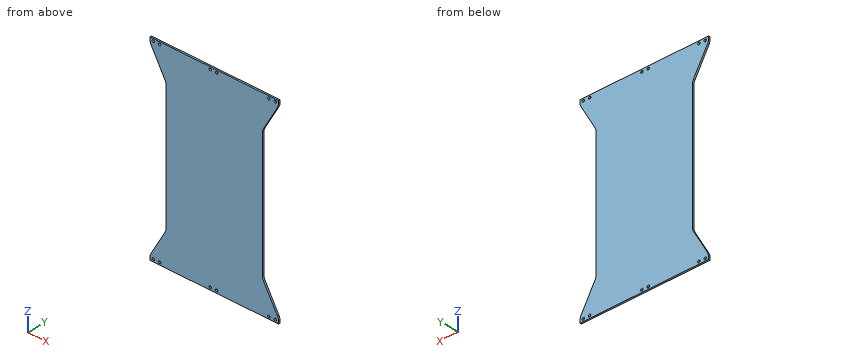
from build123d import *

# Parameters (mm, degrees)
SKETCH2_R           = 1.5
BOSS_EXTRUDE1_DEPTH = 2
FILLET1_R           = 10


with BuildPart() as part:
    # Sketch2 → Boss-Extrude1 (new body)
    with BuildSketch(Plane(origin=(0, 0, 0), x_dir=(1, 0, 0), z_dir=(0, 1, 0))):
        Polygon((688.047893911, -1476.918579287), (688.047893911, -1482.918579287), (708.047893911, -1517.918579287), (708.047893911, -1677.918579287), (688.047893911, -1712.918579287), (688.047893911, -1718.918579287), (847.682893911, -1718.918579287), (847.682893911, -1712.918579287), (827.682893911, -1677.918579287), (827.682893911, -1517.918579287), (847.682893911, -1482.918579287), (847.682893911, -1476.918579287), align=None)
        with Locations(Location((843.682893911, -1479.918579287, 0), (0, 0, 270))):
            Circle(SKETCH2_R, mode=Mode.SUBTRACT)
        with Locations(Location((835.682893911, -1479.918579287, 0), (0, 0, 270))):
            Circle(SKETCH2_R, mode=Mode.SUBTRACT)
        with Locations(Location((762.867893911, -1479.918579287, 0), (0, 0, 270))):
            Circle(SKETCH2_R, mode=Mode.SUBTRACT)
        with Locations(Location((770.867893911, -1479.918579287, 0), (0, 0, 270))):
            Circle(SKETCH2_R, mode=Mode.SUBTRACT)
        with Locations(Location((700.047893911, -1479.918579287, 0), (0, 0, 270))):
            Circle(SKETCH2_R, mode=Mode.SUBTRACT)
        with Locations(Location((692.047893911, -1479.918579287, 0), (0, 0, 270))):
            Circle(SKETCH2_R, mode=Mode.SUBTRACT)
        with Locations(Location((692.047893911, -1715.918579287, 0), (0, 0, 90))):
            Circle(SKETCH2_R, mode=Mode.SUBTRACT)
        with Locations(Location((700.047893911, -1715.918579287, 0), (0, 0, 90))):
            Circle(SKETCH2_R, mode=Mode.SUBTRACT)
        with Locations(Location((770.867893911, -1715.918579287, 0), (0, 0, 90))):
            Circle(SKETCH2_R, mode=Mode.SUBTRACT)
        with Locations(Location((762.867893911, -1715.918579287, 0), (0, 0, 90))):
            Circle(SKETCH2_R, mode=Mode.SUBTRACT)
        with Locations(Location((835.682893911, -1715.918579287, 0), (0, 0, 90))):
            Circle(SKETCH2_R, mode=Mode.SUBTRACT)
        with Locations(Location((843.682893911, -1715.918579287, 0), (0, 0, 90))):
            Circle(SKETCH2_R, mode=Mode.SUBTRACT)
    extrude(amount=BOSS_EXTRUDE1_DEPTH)

    # Fillet1
    fillet1_edges = [part.edges().sort_by_distance(p)[0] for p in [
        (847.682893911, 1, 1712.918579287),
        (688.047893911, 1, 1712.918579287),
        (708.047893911, 1, 1677.918579287),
        (708.047893911, 1, 1517.918579287),
        (688.047893911, 1, 1482.918579287),
        (847.682893911, 1, 1482.918579287),
        (827.682893911, 1, 1517.918579287),
        (827.682893911, 1, 1677.918579287),
    ]]
    fillet(fillet1_edges, radius=FILLET1_R)


solid = part.part
Source: CAD feature listing. Evaluate the final solid. Frame: model axes, mm. Round coordinates to 2 decimals unless told otherwise and drop trailing zeros. Loops run counter-clockwise (first coordinate to the right, second up) from the corner with the lowest first, then second, coordinate; pieces in that order, holes last.
Q1. Ray query, line 1 (Z direction, x = 837, y = 1.6); line 2 (Z direction, x = 771.5, y = 0.2); line 3 (X direction, y = 0.6, z = 1610). Return the intervals inside material, ascending.
Q2. Section B-B, the plane z = 1660.5. Return loops of the section in (x, y), plus the area to 3 significant figures.
Q3. Section A-A, the plane y = 0.7. State how many separate pieces and enclosed holes the cut face has, plus the area to 3 significant figures.
Q4. First-contact query: P1, Ø3.5, axis at x = 843.68, z = 1715.92, coming from the +Y side; P2, Ø2.5, axis at x = 770.87, z = 1715.92, coming from the -Y side. Flat tips, straight axial feed; report the tip coordinate or a pass-through.
Solutions:
1. line 1: z = 1476.92 to 1479.2, 1480.64 to 1501.61, 1694.22 to 1715.2, 1716.64 to 1718.92
1. line 2: z = 1476.92 to 1478.56, 1481.28 to 1714.56, 1717.28 to 1718.92
1. line 3: x = 708.05 to 827.68
2. outline: (708.05, 0) - (827.68, 0) - (827.68, 2) - (708.05, 2) - close
2. area: 239 mm2
3. separate pieces: 1
3. enclosed holes: 12
3. area: 30,700 mm2
4. P1: stops at y = 2
4. P2: passes through
